from build123d import *

# Parameters (mm, degrees)
F0_W      = 6.35
F0_H      = 28.575
F1_DEPTH  = 14.224
F4_DEPTH  = 130.049
F6_W      = 73.406
F6_H      = 6.35
F7_DEPTH  = 48.387
F9_W      = 73.406
F9_H      = 6.35
F10_DEPTH = 53.975


with BuildPart() as f1:
    # F0 (on Front) → F1 (new body, symmetric)
    with BuildSketch(Plane.XZ):
        with Locations((-49.149, 30.1625)):
            Rectangle(F0_W, F0_H)
        Polygon((17.272, 44.45), (-45.974, 44.45), (-45.974, 15.875), (21.082, 15.875), (23.749, 15.875), (34.798, 26.924), (17.272, 26.924), align=None)
        with BuildLine():
            ThreePointArc((-22.098, 24.638), (-27.686, 30.226), (-22.098, 35.814))
            Line((-22.098, 35.814), (1.778, 35.814))
            ThreePointArc((1.778, 35.814), (7.366, 30.226), (1.778, 24.638))
            Line((1.778, 24.638), (-22.098, 24.638))
        make_face(mode=Mode.SUBTRACT)
        Polygon((-45.974, 15.875), (-52.324, 15.875), (-52.324, -15.875), (-45.974, -15.875), (21.082, -15.875), (21.082, 15.875), align=None)
        Polygon((52.324, 44.45), (17.272, 44.45), (17.272, 26.924), (34.798, 26.924), align=None)
        with Locations((-49.149, -30.1625)):
            Rectangle(F0_W, F0_H)
        Polygon((21.082, -15.875), (-45.974, -15.875), (-45.974, -44.45), (17.272, -44.45), (17.272, -26.924), (34.798, -26.924), (23.749, -15.875), align=None)
        with BuildLine():
            Line((1.778, -35.814), (-22.098, -35.814))
            ThreePointArc((-22.098, -35.814), (-27.686, -30.226), (-22.098, -24.638))
            Line((-22.098, -24.638), (1.778, -24.638))
            ThreePointArc((1.778, -24.638), (7.366, -30.226), (1.778, -35.814))
        make_face(mode=Mode.SUBTRACT)
        Polygon((17.272, -26.924), (17.272, -44.45), (52.324, -44.45), (34.798, -26.924), align=None)
    extrude(amount=F1_DEPTH, both=True)

    # F3 (on offset) → F4 (cut, through all)
    with BuildSketch(Plane(origin=(-77.724, 0, 0), x_dir=(0, -1, 0), z_dir=(-1, 0, 0))):
        Polygon((-14.224, 44.45), (-14.224, 15.875), (-7.874, 15.875), (-7.874, 26.924), (-12.7, 26.924), (-12.7, 44.45), align=None)
        Polygon((7.874, 26.924), (7.874, 15.875), (14.224, 15.875), (14.224, 44.45), (12.7, 44.45), (12.7, 26.924), align=None)
        Polygon((-7.874, -15.875), (-14.224, -15.875), (-14.224, -44.45), (-12.7, -44.45), (-12.7, -26.924), (-7.874, -26.924), align=None)
        Polygon((14.224, -15.875), (7.874, -15.875), (7.874, -26.924), (12.7, -26.924), (12.7, -44.45), (14.224, -44.45), align=None)
    extrude(amount=-F4_DEPTH, mode=Mode.SUBTRACT)

    # F6 (on offset) → F7 (cut, through all)
    with BuildSketch(Plane.XY.offset(64.262)):
        Polygon((-52.324, -14.224), (21.082, -14.224), (21.082, -7.874), (-45.974, -7.874), (-45.974, -3.048), (-52.324, -3.048), align=None)
        with Locations((-15.621, 11.049)):
            Rectangle(F6_W, F6_H)
    extrude(amount=-F7_DEPTH, mode=Mode.SUBTRACT)

    # F9 (on offset) → F10 (cut, through all)
    with BuildSketch(Plane(origin=(0, 0, -69.85), x_dir=(1, 0, 0), z_dir=(0, 0, -1))):
        Polygon((-52.324, 14.224), (-52.324, 3.048), (-45.974, 3.048), (-45.974, 7.874), (21.082, 7.874), (21.082, 14.224), align=None)
        with Locations((-15.621, -11.049)):
            Rectangle(F9_W, F9_H)
    extrude(amount=-F10_DEPTH, mode=Mode.SUBTRACT)


solid = f1.part
Geometry: final body of the model. Coordinates: model frame, mm. A direction names the side the tool comes from. Round coordinates to 2 decimals unless told otherwise and drop trailing zeros. Loops run counter-clockwise (first coordinate to the right, second up) from the corner with the lowest first, then second, coordinate; pieces in that order, holes last.
Q1. Material intervals for L1, parallel to Z at x = -20.5, y = 3.25; L2, parallel to Z at x = 25, y = 11.75; L3, parallel to X at y = -7, z = 6, sorted ascending.
Q2. Section A-A on y = -9. Return loops of the section in (x, z) (3 decimals).
Q3. Access query for faces 1 (the flat face through (-10, 0, -24.638)), 2 (the flat face through (41.412, -0.178, -33.538)), 3 (the flat face through (33, 12.7, -38)), 4 (the flat face through (-49, -3.048, -30)), 5 (the flat face through (28, -10, 26.924)). Directions: +Z, -Z, +X, -X, +Y, -Y. A direction counts if a zero-diameter tool reaches every point of the face in a straight line with its end or side. Return the directions, or none.
Q4. Section D-D on z = 29. Return loops of the section in (x, y), plus the area to 3 significant figures.
Q5. Pull-direction query (Z, two-part tool) for faces 6 (the flat face through (12, 0, 44.45)), 7 (the flat face through (-16, -14.224, 0)), 8 (the flat face through (22, 0, -15.875)); classes: released by +Z, released by -Z, zero draft, split by the parting line, or undercut.
Q6. Pin query (flat end, axial travel): P1, Ø6, axis at y = 8.5, z = -15.5, coming from the +X side; P2, Ø1, axis at x = -14.5, z = 20.5, coming from the -Y side; P3, Ø2, axis at y = -10.5, z = -18, coming from the +X side; P4, Ø5, axis at x = 2, z = -18.5, coming from the +Y side. Return the tip coordinate at first contact, or that it passes through.
Q7. Section C-C on x = -32. Return loops of the section in (y, z) (3 decimals), plus the area to 3 significant figures.
Q8. Section B-B on x = -17. Return loops of the section in (y, z) (3 decimals), plus the area to 3 significant figures.
Evaluation:
1. L1: z = -44.45 to -35.81, -24.64 to 24.64, 35.81 to 44.45
1. L2: z = -44.45 to -26.92, 26.92 to 44.45
1. L3: x = -52.32 to 21.08
2. outline: (-52.324, -15.875) - (21.082, -15.875) - (21.082, 15.875) - (-52.324, 15.875) - close; (21.082, -44.45) - (52.324, -44.45) - (34.798, -26.924) - (21.082, -26.924) - close; (21.082, 26.924) - (34.798, 26.924) - (52.324, 44.45) - (21.082, 44.45) - close
3. face 1: +Y, -Y
3. face 2: +X, +Y, -Y
3. face 3: +Z, -Z, +X, -X, +Y
3. face 4: -Z, -X, -Y
3. face 5: +X, -X, -Y
4. outline: (-52.32, -3.05) - (-45.97, -3.05) - (-45.97, -7.87) - (-27.55, -7.87) - (-27.55, 7.87) - (-52.32, 7.87) - close; (7.23, -7.87) - (21.08, -7.87) - (21.08, -12.7) - (36.87, -12.7) - (36.87, 12.7) - (21.08, 12.7) - (21.08, 7.87) - (7.23, 7.87) - close
4. area: 979 mm2
5. face 6: released by +Z
5. face 7: zero draft
5. face 8: undercut
6. P1: stops at x = 26.31
6. P2: stops at y = -7.87
6. P3: passes through
6. P4: stops at y = 7.87
7. outline: (-14.224, -15.875) - (-7.874, -15.875) - (-7.874, -44.45) - (7.874, -44.45) - (7.874, -15.875) - (14.224, -15.875) - (14.224, 15.875) - (7.874, 15.875) - (7.874, 44.45) - (-7.874, 44.45) - (-7.874, 15.875) - (-14.224, 15.875) - close
7. area: 1,800 mm2
8. outline: (-14.224, -15.875) - (-7.874, -15.875) - (-7.874, -24.638) - (7.874, -24.638) - (7.874, -15.875) - (14.224, -15.875) - (14.224, 15.875) - (7.874, 15.875) - (7.874, 24.638) - (-7.874, 24.638) - (-7.874, 15.875) - (-14.224, 15.875) - close; (-7.874, -44.45) - (7.874, -44.45) - (7.874, -35.814) - (-7.874, -35.814) - close; (-7.874, 35.814) - (7.874, 35.814) - (7.874, 44.45) - (-7.874, 44.45) - close
8. area: 1,450 mm2
